Source: CAD feature listing. Evaluate the final solid. Frame: model axes, mm. A direction names the side the tool comes from. Give positions to 0.01 mm unless a question says otherwise; leave off trailing zeros. Order: outer loops, then holes, each group sorted by start corner. A loop starts at its lowest first (then second) coordinate and runs counter-clockwise, first axis right, second up. Notation, with made-up numbers: (-9, -14.5) -> (3, -14.5) arc R18 cw to (3, -3.5) -> close; hole circle Ø4 at (-14, -9). An arc over 180 degrees is marked (long way). Answer in a Markdown table with one row per item.
```python
from build123d import *

# Parameters (mm, degrees)
F4_D           = 5
F4_DEPTH       = 18
F4_TIP         = 1.5021515476
F4_ON_F3_D     = 5
F4_ON_F3_DEPTH = 18
F4_ON_F3_TIP   = 1.5021515476
F5_SIZE        = 1
F8_DEPTH       = 4


with BuildPart() as f1:
    # F0 (on Right) → F1 (revolve)
    with BuildSketch(Plane.YZ):
        Polygon((-87.5, 12.5), (-87.5, 0), (87.5, 0), (87.5, 12.5), (62.5, 12.5), (62.5, 15), (32.5, 15), (32.5, 12.5), align=None)
    revolve(axis=Axis((0, 0, 0), (0, 1, 0)))

    # F4
    with Locations(Plane.XZ.offset(87.5)):
        with Locations((0, 0)):
            Hole(F4_D / 2, depth=F4_DEPTH)
            with Locations((0, 0, -(F4_DEPTH + F4_TIP / 2))):  # 118° drill point
                Cone(0, F4_D / 2, F4_TIP, mode=Mode.SUBTRACT)

    # F4 on F3
    with Locations(Plane(origin=(0, 87.5, 0), x_dir=(-1, 0, 0), z_dir=(0, 1, 0))):
        with Locations((0, 0)):
            Hole(F4_ON_F3_D / 2, depth=F4_ON_F3_DEPTH)
            with Locations((0, 0, -(F4_ON_F3_DEPTH + F4_ON_F3_TIP / 2))):  # 118° drill point
                Cone(0, F4_ON_F3_D / 2, F4_ON_F3_TIP, mode=Mode.SUBTRACT)

    # F5
    f5_edges = [f1.edges().sort_by_distance(p)[0] for p in [
        (0, -87.5, -12.5),
        (0, 87.5, -12.5),
        (0, 32.5, -15),
        (0, 62.5, -15),
    ]]
    chamfer(f5_edges, length=F5_SIZE)

    # F7 (on offset) → F8 (cut)
    with BuildSketch(Plane.XY.offset(12.5)):
        with BuildLine():
            ThreePointArc((-4, -77.5), (0, -81.5), (4, -77.5))
            Line((4, -77.5), (4, 22.5))
            ThreePointArc((4, 22.5), (0, 26.5), (-4, 22.5))
            Line((-4, 22.5), (-4, -77.5))
        make_face()
        with BuildLine():
            ThreePointArc((-4, 67.5), (0, 63.5), (4, 67.5))
            Line((4, 67.5), (4, 82.5))
            ThreePointArc((4, 82.5), (0, 86.5), (-4, 82.5))
            Line((-4, 82.5), (-4, 67.5))
        make_face()
    extrude(amount=-F8_DEPTH, mode=Mode.SUBTRACT)


solid = f1.part
```
(1) Section query B-B (y = 55.5). Return the cut outline in (x, z), plus the area to 3 significant figures.
A:
| item | result |
|---|---|
| outline | circle Ø30 at (0, 0) |
| area | 707 mm^2 |
(2) Section query C-C (y = -49). Return the cut outline in (x, z).
A:
| item | result |
|---|---|
| outline | (-4, 8.5) -> (-4, 11.84) arc R12.5 ccw (long way) to (4, 11.84) -> (4, 8.5) -> close |
(3) Pull-direction query (Y, two-part tool) for faces 1 (the flat face through (-4, -27, 10)), 2 (the conical face through (0, -68, 0)), 3 (the flat face through (11.5, 62.5, 5.3)); classes: +Y half, -Y half, draft (parallel to the pull), parting line (faces both ways), or undercut.
A:
| item | result |
|---|---|
| face 1 | undercut |
| face 2 | -Y half |
| face 3 | +Y half |
(4) First-contact query: pin 1 Ø1.7 at (y, z) = (-49.5, 10.5) entering from -X; pin 2 Ø12 at (x, y) = (5.5, -20.5) entering from +Z; pin 3 Ø3 at (y, z) = (-57.5, 7.5) entering from -X. Flat tips, straight axial feed; report the tip coordinate or a pass-through.
A:
| item | result |
|---|---|
| pin 1 | stops at x = -7.95 |
| pin 2 | stops at z = 11.84 |
| pin 3 | stops at x = -10.97 |
(5) Section query A-A (y = -73). Return the cut outline in (x, z), plus the area to 3 significant figures.
A:
| item | result |
|---|---|
| outline | (-4, 8.5) -> (-4, 11.84) arc R12.5 ccw (long way) to (4, 11.84) -> (4, 8.5) -> close; hole circle Ø5 at (0, 0) |
| area | 441 mm^2 |
(6) Ray query, probe 1 along X at (y, z) = (-74, 0); probe 2 along Y at (x, z) = (13.25, -4); probe 3 along Z at (x, y) = (7.25, -61.5). Return the intervals inside material, ascending.
A:
| item | result |
|---|---|
| probe 1 | x = -12.5 to -2.5, 2.5 to 12.5 |
| probe 2 | y = 32.5 to 62.5 |
| probe 3 | z = -10.18 to 10.18 |
(7) Access query for faces 4 (the flat face through (0, -87.5, -3)), 5 (the flat face through (-4, 75, 10)), 6 (the flat face through (11.5, 32.5, -5.3)), 7 (the flat face through (0, 87.5, 3)), 8 (the cylindrical face through (-7.606, 74.332, -9.92)). Directions: +Z, -Z, +X, -X, +Y, -Y. A direction counts if a zero-diameter tool reaches every point of the face in a straight line with its end or side. Return the directions, or none.
A:
| item | result |
|---|---|
| face 4 | +Z, -Z, +X, -X, -Y |
| face 5 | +Z |
| face 6 | -Y |
| face 7 | +Z, -Z, +X, -X, +Y |
| face 8 | +Y |
